from build123d import *

# Parameters (mm, degrees)
SKETCH1_R           = 6
BOSS_EXTRUDE1_DEPTH = 4
SKETCH2_R           = 4
BOSS_EXTRUDE2_DEPTH = 29
SKETCH3_R           = 2.5
BOSS_EXTRUDE3_DEPTH = 7
CHAMFER1_SIZE       = 0.5
CHAMFER2_SIZE       = 1
SKETCH4_R           = 2.5
CUT_EXTRUDE1_DEPTH  = 1
FILLET1_R           = 0.5
SCALE1_SCALE        = 0.5


with BuildPart() as part:
    # Sketch1 → Boss-Extrude1 (new body)
    with BuildSketch(Plane(origin=(0, 0, 0), x_dir=(0, 0, -1), z_dir=(1, 0, 0))):
        Circle(SKETCH1_R)
    extrude(amount=BOSS_EXTRUDE1_DEPTH)

    # Sketch2 → Boss-Extrude2 (add)
    with BuildSketch(Plane(origin=(4, 0, 0), x_dir=(0, 0, -1), z_dir=(1, 0, 0))):
        Circle(SKETCH2_R)
    extrude(amount=BOSS_EXTRUDE2_DEPTH)

    # Sketch3 → Boss-Extrude3 (add)
    with BuildSketch(Plane(origin=(33, 0, 0), x_dir=(0, 0, -1), z_dir=(1, 0, 0))):
        Circle(SKETCH3_R)
    extrude(amount=BOSS_EXTRUDE3_DEPTH)

    # Chamfer1
    chamfer1_edges = [part.edges().sort_by_distance(p)[0] for p in [
        (40, 0, 2.5),
    ]]
    chamfer(chamfer1_edges, length=CHAMFER1_SIZE)

    # Chamfer2
    chamfer2_edges = [part.edges().sort_by_distance(p)[0] for p in [
        (0, 0, 6),
    ]]
    chamfer(chamfer2_edges, length=CHAMFER2_SIZE)

    # Sketch4 → Cut-Extrude1 (cut)
    with BuildSketch(Plane.ZY):
        Circle(SKETCH4_R)
    extrude(amount=-CUT_EXTRUDE1_DEPTH, mode=Mode.SUBTRACT)

    # Fillet1
    fillet1_edges = [part.edges().sort_by_distance(p)[0] for p in [
        (0, 0, -2.5),
    ]]
    fillet(fillet1_edges, radius=FILLET1_R)


with BuildPart() as part_1:
    # Scale1: scaled about (0, 0, 0)
    add(part.part.scale(SCALE1_SCALE))


solid = part_1.part
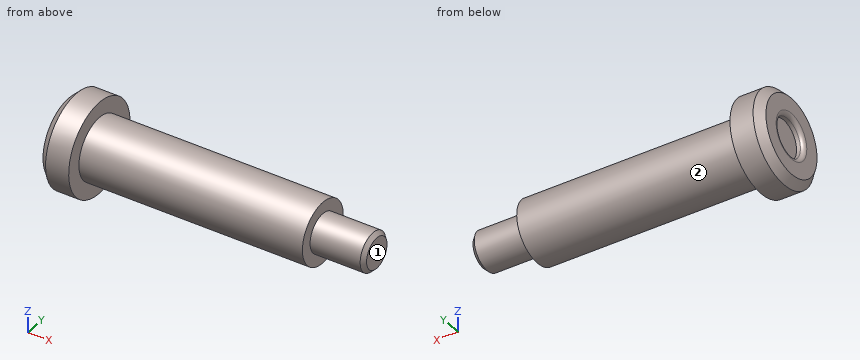
Work out the finished part from the listing and answer in its coordinate system (mm). Face numbers are marked on the shaded views. A direction names the side the tool comes from. Round coordinates to 2 decimals unless told otherwise and drop trailing zeros. Order: outer loops, then holes, each group sorted by start corner. A loop starts at its lowest first (then second) coordinate and runs counter-clockwise, first axis right, second up. Notation, with made-up numbers: M 86,9.5 L 108,9.5 A11 ccw 108,30.5 Z; hole C -11.5,37.25 d3. An arc over 180 degrees is marked long. One line per item, written item: value.
Q1. For the marked faces 1 and 2, determine the directions among +Z, -Z, +X, -X, +Y, -Y from which every point of the face is accessible in a straight line to the end or side of a thin tool.
Derived:
face 1: +Z, -Z, +X, +Y, -Y
face 2: +X
Q2. Find section D-D on x = 13. Write down the section's boundary in (y, z).
Derived:
outline: C 0,0 d4
Q3. Straight lines are drawn through the part: line 1 (X direction, y = -0.5, z = 0.8); line 2 (Y direction, x = 0.4, z = 0); line 3 (X direction, y = 0, z = -2.2). For each, find the intervals that lie inside material, in ascending order.
Derived:
line 1: 0.5 to 20
line 2: -2.9 to -1.25, 1.25 to 2.9
line 3: 0 to 2
Q4. Find section C-C on x = 18.5. Write down the section's boundary in (y, z).
Derived:
outline: C 0,0 d2.5
Q5. Find section A-A on y = 0. Write down the section's boundary in (x, z).
Derived:
outline: M 0,-2.5 L 0.5,-3 L 2,-3 L 2,-2 L 16.5,-2 L 16.5,-1.25 L 19.75,-1.25 L 20,-1 L 20,1 L 19.75,1.25 L 16.5,1.25 L 16.5,2 L 2,2 L 2,3 L 0.5,3 L 0,2.5 L 0,1.5 A0.25 ccw 0.25,1.25 L 0.5,1.25 L 0.5,-1.25 L 0.25,-1.25 A0.25 ccw 0,-1.5 Z
Q6. Flat-ended cylindrical pins translate along their axes: pin 1 (0.8 mm diameter, centred on y = 0.5, z = 0, fed in from -X); pin 2 (1.5 mm diameter, centred on x = 12.5, y = -0.5, fed in from -Z); pin 3 (3 mm diameter, centred on x = 7, y = -1.5, fed in from +Z). Find the tip coordinate at first contact, or state that the pin passes through.
Derived:
pin 1: x = 0.5
pin 2: z = -2
pin 3: z = 2
